Source: three-view drawing plus pictorial views. Frame: mm from the lowest corner of the part. A direction names the side the tool comes from. Give positions to 0.01 mm unless a question says otherwise; leave off trailing zeros. Order: outer loops, then holes, each group sorted by start corner. A loop starts at its lowest first (then second) coordinate and runs counter-clockwise, first axis right, second up. Notation, with made-up numbers: M 18,66.5 L 30,66.5 A21 cw 30,96.5 Z; hole C 12.5,85.5 d7. An arc over 180 degrees is marked long. Use CSV: the item, a comma, the result in double quotes. Start each with the question number.
Item 1: Section query C-C on y = 29. Return loops of the section in (x, z), and give its area (3 significant figures).
Item 2: Pull-direction query (Y, two-part tool) for the marked faces 1, 2 and 3; classes: +Y half, -Y half, draft (parallel to the pull), parting line (faces both ways), or undercut.
Item 3: Access query for the marked faces 4, 5, 6 and 7. Directions: +Z, -Z, +X, -X, +Y, -Y. A direction counts if a zero-diameter tool reaches every point of the face in a straight line with its end or side. Return the directions, or none.
Item 4: First-contact query: pin 1 (1 mm diameter, centred on y = 7, z = 4, fed in from +X); pin 2 (9 mm diameter, centred on y = 8, z = 8, fed in from -X); pin 3 (10 mm diameter, centred on x = 17.5, y = 14, fed in from -Z); pin 4 (2.5 mm diameter, centred on x = 2.5, z = 5, fed in from -Y). Flat tips, straight axial feed; report the tip coordinate or a pass-through.
Item 5: Section query B-B on z = 10. Return loops of the section in (x, y), and give its area (3 significant figures).
Item 6: Section query D-D on x = 36.5. Return loops of the section in (y, z).
Item 7: Ray query, probe 1 along X at (y, z) = (28.85, 5); probe 2 along Y at (x, z) = (41.5, 3.25); probe 3 along Z at (x, y) = (49, 29). Return the intervals inside material, ascending. Write a range as from..to.
Item 8: Section query A-A on x = 49.5. Return loops of the section in (y, z).
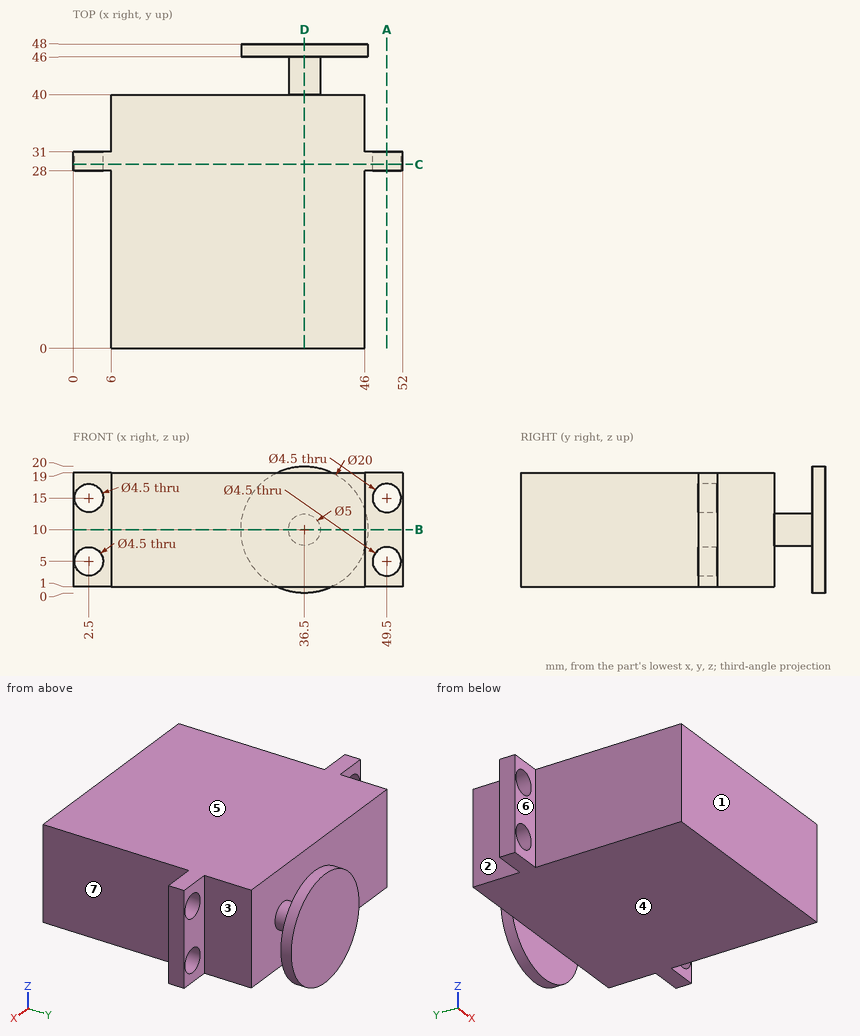
Verdict:
1,outline,"M 0,1 L 52,1 L 52,19 L 0,19 Z; hole C 2.5,5 d4.5; hole C 2.5,15 d4.5; hole C 49.5,5 d4.5; hole C 49.5,15 d4.5"
1,area,"872 mm2"
2,face 1,"-Y half"
2,face 2,"draft"
2,face 3,"undercut"
3,face 4,"-Z, +X, -X, -Y"
3,face 5,"+Z, +X, -X, -Y"
3,face 6,"+Z, -Z, -X, -Y"
3,face 7,"+Z, -Z, +X, -Y"
4,pin 1,"x = 46"
4,pin 2,"x = 6"
4,pin 3,"z = 1"
4,pin 4,"through"
5,outline,"M 0,28 L 6,28 L 6,0 L 46,0 L 46,28 L 52,28 L 52,31 L 46,31 L 46,40 L 39,40 L 39,46 L 46.5,46 L 46.5,48 L 26.5,48 L 26.5,46 L 34,46 L 34,40 L 6,40 L 6,31 L 0,31 Z"
5,area,"1,710 mm2"
6,outline,"M 0,1 L 40,1 L 40,7.5 L 46,7.5 L 46,0 L 48,0 L 48,20 L 46,20 L 46,12.5 L 40,12.5 L 40,19 L 0,19 Z"
7,probe 1,"0..0.25, 4.75..47.25, 51.75..52"
7,probe 2,"0..40, 46..48"
7,probe 3,"1..2.81, 7.19..12.81, 17.19..19"
8,outline,"M 28,1 L 31,1 L 31,2.75 L 28,2.75 Z; M 28,7.25 L 31,7.25 L 31,12.75 L 28,12.75 Z; M 28,17.25 L 31,17.25 L 31,19 L 28,19 Z"
